Geometry check sheet. Reference: the model listing, model coordinates, mm. A direction names the side the tool comes from. Give positions to 0.01 mm unless a question says otherwise; leave off trailing zeros. Loops run counter-clockwise (first coordinate to the right, second up) from the corner with the lowest first, then second, coordinate; pieces in that order, holes last. Notation, with made-up numbers: (56, 15.25) - (89, 15.25) arc R22 cw to (89, 48.25) - close; hole circle Ø1 at (3.25, 53). An arc over 180 degrees is marked (long way). Use a Markdown table: item, result. Add a question column.
1. Depth check by flat-ended pin: P1, Ø0.9, axis at y = 16.5, z = 12, coming from the +X side; P2, Ø2.5, axis at x = -13.5, z = -10, coming from the +Y side; P3, Ø12, axis at x = -4, z = 0.5, coming from the +Y side. Enter the tip coordinate at first touch or a pass-through.
2. Material ranges on L1, parallel to X at y = 16.6, z = -10 (3 decimals); L2, parallel to Z at x = -13.5, y = 16.45 (3 decimals); L3, parallel to X at y = 14.5, z = -5, recorded low to high.
3. Cross-section at D-D on x = -9. Enter the section's corners in (y, z), and give its area (3 significant figures).
4. Cross-section at C-C on y = 12. Enter the section's corners in (x, z).
5. Set-up check for faces 4 (the cylindrical face through (-15.65, 9.89, 12.18)), 5 (the flat face through (6.2, 11.2, -0.1)), 6 (the flat face through (-6, 12, 0)), 7 (the flat face through (0, 14.8, 12)), 8 (the cylindrical face through (14.27, 16.79, 8.8)): record each of +Z, -Z, +X, -X, +Y, -Y from which the full face is reachable in a straight line by a thin tool's end or side.
6. Cross-section at B-B on x = -4.5. Enter the section's corners in (y, z).
7. Draft check along Y on faces 1 (the flat face through (0, 11, -7.1)), 2 (the flat face through (-4, 16.6, 11.8)), 3 (the flat face through (-14, 14, -10)). Enter one of: pulls with the +Y half, pulls with the -Y half, needs draft (parallel to the pull), parting line crosses it, or undercut.
8. Cross-section at A-A on z = 2. Enter the section's corners in (x, y), and give its area (3 significant figures).
from build123d import *

# Parameters (mm, degrees)
SKETCH_1_W          = 32.5
SKETCH_1_H          = 25.5
SKETCH_1_W_2        = 28.5
SKETCH_1_H_2        = 21.5
EXTRUDE_1_DEPTH     = 13.2
SKETCH_2_W          = 28.5
SKETCH_2_H          = 21.5
SKETCH_2_W_2        = 12
SKETCH_2_H_2        = 12
EXTRUDE_2_DEPTH     = 2
EXTRUDE_3_DEPTH     = 6.3
EXTRUDE_4_REACH     = 21.5
SKETCH_6_R          = 2.7
SKETCH_7_R          = 1.425
CUT_EXTRUDE_3_DEPTH = 5.5
SKETCH_10_W         = 15.8
SKETCH_10_H         = 15.8
SKETCH_10_W_2       = 14.2
SKETCH_10_H_2       = 14.2
EXTRUDE_5_DEPTH     = 0.8
CUT_EXTRUDE_5_DEPTH = 3
FILLET_6_R          = 0.5
FILLET_3_R          = 0.95
FILLET_1_R          = 2
FILLET_2_R          = 1


with BuildPart() as part:
    # 草图1 → 凸台-拉伸1 (new body)
    with BuildSketch(Plane(origin=(0, 0, 0), x_dir=(1, 0, 0), z_dir=(0, 1, 0))):
        Rectangle(SKETCH_1_W, SKETCH_1_H)
        Rectangle(SKETCH_1_W_2, SKETCH_1_H_2, mode=Mode.SUBTRACT)
    extrude(amount=EXTRUDE_1_DEPTH)

    # 草图2 → 凸台-拉伸2 (add)
    with BuildSketch(Plane(origin=(0, 13.2, 0), x_dir=(1, 0, 0), z_dir=(0, 1, 0))):
        Rectangle(SKETCH_2_W, SKETCH_2_H)
        Rectangle(SKETCH_2_W_2, SKETCH_2_H_2, mode=Mode.SUBTRACT)
    extrude(amount=-EXTRUDE_2_DEPTH)

    # 草图3 → 凸台-拉伸3 (add)
    with BuildSketch(Plane(origin=(0, 13.2, 0), x_dir=(1, 0, 0), z_dir=(0, 1, 0))):
        Polygon((-16.25, -12.75), (-16.25, 12.75), (16.25, 12.75), (16.25, -0.040360215), (16.25, -12.75), align=None)
        Polygon((14.25, 0.013681835), (14.25, 10.75), (-14.25, 10.75), (-14.25, -10.75), (14.25, -10.75), align=None, mode=Mode.SUBTRACT)
    extrude(amount=EXTRUDE_3_DEPTH)

    # 草图6 → 凸台-拉伸4 (add, up to next)
    with BuildSketch(Plane(origin=(0, 19.5, 0), x_dir=(1, 0, 0), z_dir=(0, 1, 0)), mode=Mode.PRIVATE) as extrude_4_sk1:
        with Locations((13.5, 10)):
            Circle(SKETCH_6_R)
    extrude_4_tool1 = extrude(extrude_4_sk1.sketch, amount=-EXTRUDE_4_REACH, mode=Mode.PRIVATE) - part.part
    add(extrude_4_tool1.solids().sort_by_distance((13.5, 19.5, -10))[0])
    # 草图6 → 凸台-拉伸4 (add, up to next)
    with BuildSketch(Plane(origin=(0, 19.5, 0), x_dir=(1, 0, 0), z_dir=(0, 1, 0)), mode=Mode.PRIVATE) as extrude_4_sk2:
        with Locations((13.5, -10)):
            Circle(SKETCH_6_R)
    extrude_4_tool2 = extrude(extrude_4_sk2.sketch, amount=-EXTRUDE_4_REACH, mode=Mode.PRIVATE) - part.part
    add(extrude_4_tool2.solids().sort_by_distance((13.5, 19.5, 10))[0])
    # 草图6 → 凸台-拉伸4 (add, up to next)
    with BuildSketch(Plane(origin=(0, 19.5, 0), x_dir=(1, 0, 0), z_dir=(0, 1, 0)), mode=Mode.PRIVATE) as extrude_4_sk3:
        with Locations((-13.5, -10)):
            Circle(SKETCH_6_R)
    extrude_4_tool3 = extrude(extrude_4_sk3.sketch, amount=-EXTRUDE_4_REACH, mode=Mode.PRIVATE) - part.part
    add(extrude_4_tool3.solids().sort_by_distance((-13.5, 19.5, 10))[0])
    # 草图6 → 凸台-拉伸4 (add, up to next)
    with BuildSketch(Plane(origin=(0, 19.5, 0), x_dir=(1, 0, 0), z_dir=(0, 1, 0)), mode=Mode.PRIVATE) as extrude_4_sk4:
        with Locations((-13.5, 10)):
            Circle(SKETCH_6_R)
    extrude_4_tool4 = extrude(extrude_4_sk4.sketch, amount=-EXTRUDE_4_REACH, mode=Mode.PRIVATE) - part.part
    add(extrude_4_tool4.solids().sort_by_distance((-13.5, 19.5, -10))[0])

    # 草图7 → 切除-拉伸3 (cut)
    with BuildSketch(Plane(origin=(0, 19.5, 0), x_dir=(1, 0, 0), z_dir=(0, 1, 0))):
        with Locations((13.5, 10)):
            Circle(SKETCH_7_R)
        with Locations((13.5, -10)):
            Circle(SKETCH_7_R)
        with Locations((-13.5, -10)):
            Circle(SKETCH_7_R)
        with Locations((-13.5, 10)):
            Circle(SKETCH_7_R)
    extrude(amount=-CUT_EXTRUDE_3_DEPTH, mode=Mode.SUBTRACT)

    # 草图10 → 凸台-拉伸5 (add)
    with BuildSketch(Plane.XZ.offset(-11.2)):
        Rectangle(SKETCH_10_W, SKETCH_10_H)
        Rectangle(SKETCH_10_W_2, SKETCH_10_H_2, mode=Mode.SUBTRACT)
    extrude(amount=EXTRUDE_5_DEPTH)

    # 草图11 → 切除-拉伸5 (cut)
    with BuildSketch(Plane.XY.offset(12.75)):
        Polygon((-4, 17.65), (4, 17.65), (4, 15.8), (3, 14.8), (-3, 14.8), (-4, 15.8), align=None)
    extrude(amount=-CUT_EXTRUDE_5_DEPTH, mode=Mode.SUBTRACT)

    # 圆角6
    fillet_6_edges = [part.edges().sort_by_distance(p)[0] for p in [
        (4, 17.65, 11.75),
        (4, 15.8, 11.75),
        (3, 14.8, 11.75),
        (-3, 14.8, 11.75),
        (-4, 15.8, 11.75),
        (-4, 17.65, 11.75),
    ]]
    fillet(fillet_6_edges, radius=FILLET_6_R)

    # 圆角3
    fillet_3_edges = [part.edges().sort_by_distance(p)[0] for p in [
        (0, 13.2, 10.75),
        (-11.590811691, 13.2, 8.090811691),
        (-14.25, 13.2, 0),
        (-11.590811691, 13.2, -8.090811691),
        (0, 13.2, -10.75),
        (11.590811691, 13.2, -8.090811691),
        (14.25, 13.2, 0),
        (11.590811691, 13.2, 8.090811691),
    ]]
    fillet(fillet_3_edges, radius=FILLET_3_R)

    # 圆角1
    fillet_1_edges = [part.edges().sort_by_distance(p)[0] for p in [
        (16.25, 9.75, 12.75),
        (-16.25, 9.75, 12.75),
        (-16.25, 9.75, -12.75),
        (16.25, 9.75, -12.75),
    ]]
    fillet(fillet_1_edges, radius=FILLET_1_R)

    # 圆角2
    fillet_2_edges = [part.edges().sort_by_distance(p)[0] for p in [
        (-14.25, 5.6, 10.75),
        (14.25, 5.6, 10.75),
        (-14.25, 5.6, -10.75),
        (14.25, 5.6, -10.75),
    ]]
    fillet(fillet_2_edges, radius=FILLET_2_R)


solid = part.part
Values found:
| question | item | result |
|---|---|---|
| 1 | P1 | stops at x = 16.08 |
| 1 | P2 | stops at y = 14 |
| 1 | P3 | stops at y = 13.2 |
| 2 | L1 | x = -16.25 to -14.925, -12.075 to -10.8, 10.8 to 12.075, 14.925 to 16.25 |
| 2 | L2 | z = -12.75 to -11.425, -8.575 to -7.3, 7.3 to 8.575, 11.425 to 12.75 |
| 2 | L3 | x = -16.25 to -14.25, 14.25 to 16.25 |
| 3 | outline | (0, -12.75) - (19.5, -12.75) - (19.5, -10.75) - (14.15, -10.75) arc R0.95 cw to (13.2, -9.8) - (13.2, 9.8) arc R0.95 cw to (14.15, 10.75) - (19.5, 10.75) - (19.5, 12.75) - (0, 12.75) - (0, 10.75) - (11.2, 10.75) - (11.2, -10.75) - (0, -10.75) - close |
| 3 | area | 121 mm2 |
| 4 | outline | (-16.25, -10.75) arc R2 ccw to (-14.25, -12.75) - (14.25, -12.75) arc R2 ccw to (16.25, -10.75) - (16.25, 10.75) arc R2 ccw to (14.25, 12.75) - (-14.25, 12.75) arc R2 ccw to (-16.25, 10.75) - close; hole (-6, -6) - (6, -6) - (6, 6) - (-6, 6) - close |
| 5 | face 4 | +Z, -X, +Y, -Y |
| 5 | face 5 | -Y |
| 5 | face 6 | +Y, -Y |
| 5 | face 7 | +Z |
| 5 | face 8 | +Y |
| 6 | outline | (0, -12.75) - (19.5, -12.75) - (19.5, -10.75) - (14.15, -10.75) arc R0.95 cw to (13.2, -9.8) - (13.2, -6) - (11.2, -6) - (11.2, -7.1) - (10.4, -7.1) - (10.4, -7.9) - (11.2, -7.9) - (11.2, -10.75) - (0, -10.75) - close; (0, 10.75) - (11.2, 10.75) - (11.2, 7.9) - (10.4, 7.9) - (10.4, 7.1) - (11.2, 7.1) - (11.2, 6) - (13.2, 6) - (13.2, 9.8) arc R0.95 cw to (14.15, 10.75) - (19.5, 10.75) - (19.5, 12.75) - (0, 12.75) - close |
| 7 | face 1 | needs draft |
| 7 | face 2 | undercut |
| 7 | face 3 | pulls with the +Y half |
| 8 | outline | (-16.25, 0) - (-14.25, 0) - (-14.25, 11.2) - (-7.9, 11.2) - (-7.9, 10.4) - (-7.1, 10.4) - (-7.1, 11.2) - (-6, 11.2) - (-6, 13.2) - (-13.3, 13.2) arc R0.95 cw to (-14.25, 14.15) - (-14.25, 19.5) - (-16.25, 19.5) - close; (6, 11.2) - (7.1, 11.2) - (7.1, 10.4) - (7.9, 10.4) - (7.9, 11.2) - (14.25, 11.2) - (14.25, 0) - (16.25, 0) - (16.25, 19.5) - (14.25, 19.5) - (14.25, 14.15) arc R0.95 cw to (13.3, 13.2) - (6, 13.2) - close |
| 8 | area | 113 mm2 |
